The listing builds one solid part. Answer for the finished solid, in the listing's coordinates (mm). A direction names the side the tool comes from. Coordinates: 2 decimals unless noted, no trailing zeros. Loops run counter-clockwise (first coordinate to the right, second up) from the corner with the lowest first, then second, coordinate; pieces in that order, holes last. Notation, with made-up numbers: (72.5, -20) - (90.5, -20) arc R22 ccw to (90.5, 16) - close; hole circle Ø1 at (31.25, -29.75). An arc over 180 degrees is marked (long way). Write each question's results on one line, items separated by ' | '. Start each with the question number.
(1) For faces 5 (the cylindrical face through (32.6, -17.2, -2.8)), 6 (the flat face through (15.875, -40, -4)), 7 (the flat face through (8, -20, -5.613)), 8 (the flat face through (31, -41.275, -3)), 9 (the flat face through (8, -39.688, -4)), determine the directions among +Z, -Z, +X, -X, +Y, -Y from which every point of the face is accessible in a straight line to the end or side of a thin tool.
(2) Find section A-A on z = -4.85. State how many separate pieces and enclosed holes the cut face has, then the cut area to 3 significant figures.
(3) Find section C-C on x = 50. Determine the outline of the cut face in (y, z) (3 decimals).
(4) Consider line 1 (X direction, y = -31, z = -4.8) (3 decimals); line 2 (X direction, y = -6, z = -4.55) (3 decimals); line 3 (X direction, y = -27.5, z = -4.4) (3 decimals). Determine where each line is inside the solid, lowest interval first. Write a range as from..to.
(5) Find section B-B on y = -13. Determine the outline of the cut face in (x, z) (3 decimals), then the cut area to 3 significant figures.
(6) Given pin 1 Ø1.6 at (y, z) = (-30, -3.5) entering from -X; pin 2 Ø1 at (x, z) = (4, -3.5) entering from +Y (3 decimals); pin 3 Ø1.7 at (y, z) = (-40, -3.5) entering from +X, each flat-ended and moving along its own axis, determine where each tip first touches the part or whether it passes through.
(7) Determine the mould class of faces 1 (the flat face through (8, -37.528, -4)), 2 (the cylindrical face through (36.39, -33.56, -2.77)), 3 (the cylindrical face through (28.556, -16.207, -2.767)), 4 (the cylindrical face through (64.765, -1.811, -2.846)) for opening direction X: released by +X, released by -X, zero draft, split by the parting line, or undercut.
Autodesk Inventor part; units mm, degrees
ref_plane "YZ Plane" through (0, 0, 0) normal (1, 0, 0) x (0, 1, 0)
ref_plane "XZ Plane" through (0, 0, 0) normal (0, 1, 0) x (-1, 0, 0)
ref_plane "XY Plane" through (0, 0, 0) normal (0, 0, 1) x (1, 0, 0)
sketch "Sketch1" plane through (0, 0, 0) normal (0, 0, 1) x (1, 0, 0)
  line L0 (0, 0) -> (66.675, 0)
  line L1 (66.675, 0) -> (66.675, -41.275)
  line L2 (66.675, -41.275) -> (0, -41.275)
  line L3 (0, -41.275) -> (0, 0)
  arc A0 (40.6531, -3.4261) -> (33.474, -33.5752) centre (46.0375, -20.6375) ccw
  arc A1 (41.8969, -7.4017) -> (36.376, -30.5868) centre (46.0375, -20.6375) ccw
  circle A2 centre (46.0375, -20.6375) radius 8.7948
  arc A3 (41.8969, -7.4017) -> (40.6531, -3.4261) centre (41.275, -5.4139) ccw
  arc A4 (33.474, -33.5752) -> (36.376, -30.5868) centre (34.925, -32.081) ccw
  dimension "d0" = 41.275
  dimension "d1" = 66.675
  dimension "d4" = 17.5895
  dimension "d5" = 20.6375
  dimension "d22" = 20.6375
  dimension "d23" = 25.4
  dimension "d24" = 31.75
  dimension "d54" = 2.0828
  dimension "d55" = 15.9512
extrude "Extrusion1" add sketch "Sketch1" against normal blind 5.6134
sketch "Sketch5" plane through (0, 0, -5.6134) normal (0, 0, -1) x (-1, 0, 0)
  line L0 (0, 0) -> (-66.675, 0)
  line L1 (-66.675, -41.275) -> (0, -41.275)
  line L2 (0, -41.275) -> (0, 0)
  line L3 (-18.8976, 0) -> (-15.875, 0)
  line L4 (-15.875, 0) -> (-15.875, -41.275)
  line L5 (-15.875, -41.275) -> (-18.8976, -41.275)
  line L6 (-18.8976, -41.275) -> (-18.8976, 0)
  line L7 (-18.8976, 0) -> (0, 0)
  line L8 (0, 0) -> (0, -3.175)
  line L9 (0, -3.175) -> (-18.8976, -3.175)
  line L10 (-18.8976, -3.175) -> (-18.8976, 0)
  line L11 (-15.875, -39.6875) -> (0, -39.6875)
  line L12 (0, -39.6875) -> (0, -37.5285)
  line L13 (0, -37.5285) -> (-15.875, -37.5285)
  line L14 (-15.875, -37.5285) -> (-15.875, -39.6875)
  dimension "d37" = 3.0226
  dimension "d38" = 15.875
  dimension "d39" = 3.175
  dimension "d43" = 1.5875
  dimension "d44" = 2.159
extrude "Extrusion5" cut sketch "Sketch5" against normal blind 3.175 contours L2 L9 L4 L0 | L4 L9 L6 L0 | L4 L1 L6 L9 | L2 L11 L4 L13
fillet "Fillet1" radius 6.35 2 edges at (66.675, 0, -2.8067) (66.675, -41.275, -2.8067)
properties part number "Lidar Sensor Case v4 Piece 3"
Values:
1) face 5: +Z, -Z | face 6: -Z, +Y, -Y | face 7: -Z, +X, -X, +Y, -Y | face 8: +Z, -Z, +X, -X, -Y | face 9: -Z, -X
2) separate pieces: 3 | enclosed holes: 2 | area: 2,130 mm²
3) outline: (-41.275, -5.613) - (-28.489, -5.613) - (-28.489, 0) - (-41.275, 0) - close; (-12.786, -5.613) - (0, -5.613) - (0, 0) - (-12.786, 0) - close
4) line 1: x = 0..15.875, 18.898..31.278, 36.705..66.675 | line 2: x = 0..15.875, 18.898..35.503, 43.274..66.665 | line 3: x = 0..15.875, 18.898..29.36, 33.986..40.537, 51.538..66.675
5) outline: (0, -5.613) - (15.875, -5.613) - (15.875, -2.438) - (18.898, -2.438) - (18.898, -5.613) - (29.701, -5.613) - (29.701, 0) - (0, 0) - close; (34.462, -5.613) - (41.677, -5.613) - (41.677, 0) - (34.462, 0) - close; (50.398, -5.613) - (66.675, -5.613) - (66.675, 0) - (50.398, 0) - close | area: 289 mm²
6) pin 1: stops at x = 0 | pin 2: stops at y = -3.175 | pin 3: stops at x = 65.07
7) face 1: zero draft | face 2: undercut | face 3: undercut | face 4: released by +X
